Job drawing, mm, ordinate dimensions from the low corner. One solid piece. Give positions to 0.01 mm unless a question says otherwise; leave off trailing zeros. Order: outer loops, then holes, each group sorted by start corner. A loop starts at its lowest first (then second) coordinate and runs counter-clockwise, first axis right, second up.
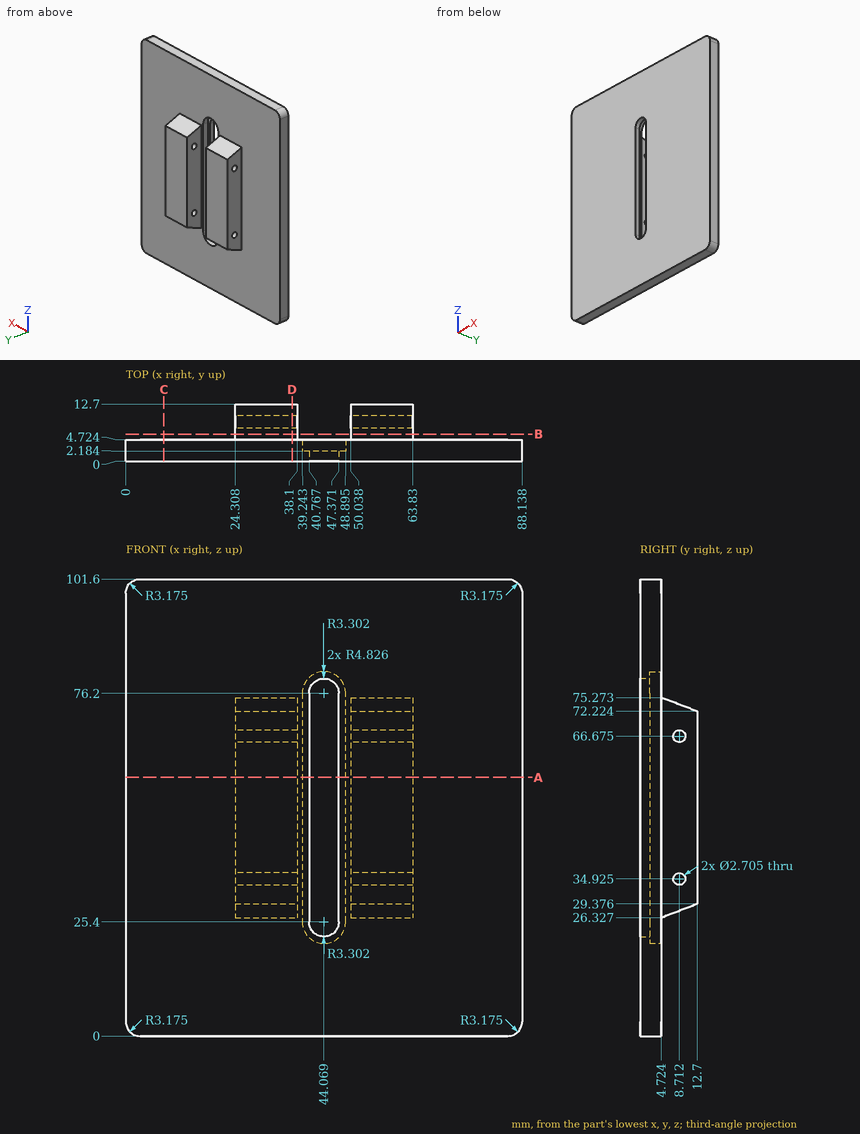
Item 1: Band-saw the part on C-C on x = 8.5. List the corners of the cut face in (y, z) (1 decimal).
Item 2: Band-saw the part on B-B on y = 6. List the corners of the cut face in (x, z) (1 decimal), plus the area to 3 significant figures.
Item 3: Band-saw the part on D-D on x = 37. List the corners of the cut face in (y, z) (1 decimal).
Item 4: Drop flat-ended pins along their axis: P1, Ø3, axis at y = 8.71, z = 66.68, coming from the +X side; P2, Ø2, axis at y = 11, z = 60.5, coming from the -X side; P3, Ø7.5, axis at x = 42, z = 58.5, coming from the +Y side. Give the stop position or say it passes through.
Item 5: Drill centre lines: probe 1 along X at (y, z) = (10, 34); probe 2 along X at (y, z) = (1, 40.5); probe 3 along Z at (x, y) = (36.5, 9). Where is each one in solid material? Low to high.
Item 6: Band-saw the part on A-A on z = 57.5. List the corners of the cut face in (x, y) (1 decimal).
Working result:
1. outline: (0, 0) - (4.7, 0) - (4.7, 101.6) - (0, 101.6) - close
2. outline: (24.3, 26.8) - (38.1, 26.8) - (38.1, 74.8) - (24.3, 74.8) - close; (50, 26.8) - (63.8, 26.8) - (63.8, 74.8) - (50, 74.8) - close
2. area: 1,320 mm2
3. outline: (0, 0) - (4.7, 0) - (4.7, 26.3) - (12.7, 29.4) - (12.7, 72.2) - (4.7, 75.3) - (4.7, 101.6) - (0, 101.6) - close; hole circle Ø2.7 at (8.7, 34.9); hole circle Ø2.7 at (8.7, 66.7)
4. P1: stops at x = 63.83
4. P2: stops at x = 24.31
4. P3: stops at y = 4.72
5. probe 1: x = 24.31 to 38.1, 50.04 to 63.83
5. probe 2: x = 0 to 40.77, 47.37 to 88.14
5. probe 3: z = 27.96 to 33.6, 36.25 to 65.35, 68 to 73.64
6. outline: (0, 0) - (40.8, 0) - (40.8, 2.2) - (39.2, 2.2) - (39.2, 4.7) - (38.1, 4.7) - (38.1, 12.7) - (24.3, 12.7) - (24.3, 4.7) - (0, 4.7) - close; (47.4, 0) - (88.1, 0) - (88.1, 4.7) - (63.8, 4.7) - (63.8, 12.7) - (50, 12.7) - (50, 4.7) - (48.9, 4.7) - (48.9, 2.2) - (47.4, 2.2) - close
